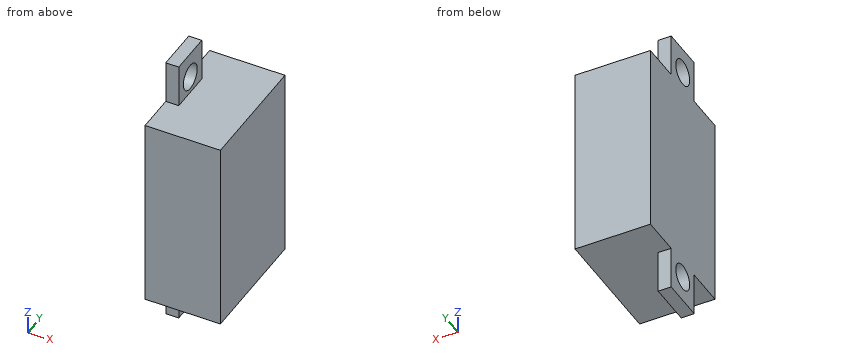
Autodesk Inventor part; units mm, degrees
ref_plane "YZ Plane" through (0, 0, 0) normal (1, 0, 0) x (0, 1, 0)
ref_plane "XZ Plane" through (0, 0, 0) normal (0, 1, 0) x (-1, 0, 0)
ref_plane "XY Plane" through (0, 0, 0) normal (0, 0, 1) x (1, 0, 0)
sketch "Sketch1" plane through (0, 0, 0) normal (1, 0, 0) x (0, 1, 0)
  line L0 (0, 0) -> (14, 0)
  line L1 (14, 0) -> (14, -22.5)
  line L2 (14, -22.5) -> (0, -22.5)
  line L3 (0, -22.5) -> (0, 0)
  dimension "d0" = 14
  dimension "d1" = 22.5
extrude "Extrusion1" add sketch "Sketch1" along normal blind 7.2
sketch "Sketch2" plane through (0, 0, 0) normal (-1, 0, 0) x (0, 0, 1)
  line L0 (-22.5, 0) -> (-22.5, 14)
  line L1 (0, 0) -> (-22.5, 0)
  line L2 (0, 14) -> (0, 0)
  line L3 (-22.5, 14) -> (0, 14)
extrude "Extrusion2" add sketch "Sketch2" along normal blind 1.5
sketch "Sketch3" plane through (7.2, 0, 0) normal (0, 0, 1) x (1, 0, 0)
  line L0 (-8.7, 0) -> (-8.7, 14)
  line L1 (-8.7, 14) -> (0, 14)
  line L2 (-8.7, 0) -> (-7.2, 0)
  line L3 (-7.2, 0) -> (-7.2, 14)
  line L4 (-7.2, 14) -> (-8.7, 14)
  line L5 (-8.7, 14) -> (-8.7, 0)
  line L6 (-8.7, 7) -> (-7.2, 7)
  line L7 (-8.7, 9.5) -> (-7.2, 9.5)
  line L8 (-7.2, 9.5) -> (-7.2, 4.5)
  line L9 (-7.2, 4.5) -> (-8.7, 4.5)
  line L10 (-8.7, 4.5) -> (-8.7, 9.5)
  line L11 (-8.7, 9.5) -> (-7.2, 4.5) construction
  line L12 (-7.2, 9.5) -> (-8.7, 4.5) construction
  point P0 (-7.95, 7)
  dimension "d6" = 5
extrude "Extrusion3" add sketch "Sketch3" along normal blind 5 contours L0 L6 L3 L9 | L0 L7 L3 L6
sketch "Sketch4" plane through (7.2, 0, -22.5) normal (0, 0, -1) x (-1, 0, 0)
  line L0 (8.7, 9.5) -> (8.7, 4.5)
  line L1 (8.7, 4.5) -> (7.2, 4.5)
  line L2 (7.2, 4.5) -> (7.2, 9.5)
  line L3 (7.2, 9.5) -> (8.7, 9.5)
  point P0 (7.2, 0)
extrude "Extrusion4" add sketch "Sketch4" along normal blind 5
sketch "Sketch5" plane through (0, 4.5, -22.5) normal (1, 0, 0) x (0, 0, -1)
  line L0 (-22.5, 5) -> (-27.5, 5)
  line L1 (-22.5, 0) -> (-27.5, 0)
  line L2 (-27.5, 0) -> (-27.5, 5)
  line L3 (0, -4.5) -> (0, 9.5)
  line L4 (-22.5, 9.5) -> (-22.5, -4.5)
  line L5 (0, 5) -> (5, 5)
  line L6 (0, 0) -> (5, 0)
  line L7 (-27.5, 2.5) -> (-22.5, 2.5)
  line L8 (0, 2.5) -> (5, 2.5)
  line L9 (-22.5, 2.5) -> (-23, 2.5)
  line L10 (0, 2.5) -> (0.5, 2.5)
  line L11 (-23, 2.5) -> (-24.5, 2.5)
  circle A0 centre (-24.5, 2.5) radius 1.5
  line L12 (0.5, 2.5) -> (2, 2.5)
  circle A1 centre (2, 2.5) radius 1.5
  dimension "d11" = 0.5
  dimension "d12" = 0.5
  dimension "d13" = 1.5
  dimension "d14" = 1.5
extrude "Extrusion5" cut sketch "Sketch5" against normal blind 5 contours A0 L7 | L7 A0 | A1 L8 | L8 A1
sketch "Sketch6" plane through (7.2, 0, 0) normal (1, 0, 0) x (0, 0, -1)
  line L0 (0, 14) -> (22.5, 14)
  line L1 (0, 14) -> (22.6011, 13.9799) construction
  line L2 (22.6011, 13.9799) -> (22.5897, 1.2087) construction
  line L3 (22.5897, 1.2087) -> (-0.0114, 1.2289) construction
  line L4 (-0.0114, 1.2289) -> (0, 14) construction
  point P0 (0, 0)
properties part number "Voltmeter"
Design review of the part built by this model. Coordinates are the model's own, in mm. Give positions to 0.01 mm unless a question says otherwise; leave off trailing zeros. Order: outer loops, then holes, each group sorted by start corner. A loop starts at its lowest first (then second) coordinate and runs counter-clockwise, first axis right, second up. Notation, with made-up numbers: (33.5, 57) - (40.5, 57) arc R23 cw to (40.5, 85) - close; hole circle Ø4 at (58.25, -31.5). An arc over 180 degrees is marked (long way). Write item = value, one per line. Start each with the question number.
Q1. To check wall thickness, follow L1, parallel to Z at x = -0.6, y = 7; L2, parallel to Y at x = -0.85, z = -24.5; L3, parallel to Z at x = 4.75, y = 13. State the ranges of each line that lie inside material, in increasing order. Write a range as from..to.
Q2. We need section B-B on z = -24.5. State the section outline as (x, y) points, plus the area to 3 significant figures.
Q3. We need section A-A on y = 7. State the section outline as (x, z) points.
Q4. Clearance check with flat-ended pins moving along their axes: pin 1 Ø2.5 at (y, z) = (7.5, 2.5) entering from +X; pin 2 Ø2.5 at (y, z) = (7, 2) entering from +X; pin 3 Ø1.2 at (x, z) = (-1, 3) entering from -Y. State where each tip first meets the part, or that it passes through.
Q5. We need section D-D on y = 1.5. State the section outline as (x, z) points.
Q6. We need section C-C on x = 6.5. State the section outline as (y, z) points.
Working result:
q1.L1 = -27.5..-26, -23..0.5, 3.5..5
q1.L2 = 4.5..5.5, 8.5..9.5
q1.L3 = -22.5..0
q2.outline = (-1.5, 4.5) - (0, 4.5) - (0, 5.5) - (-1.5, 5.5) - close; (-1.5, 8.5) - (0, 8.5) - (0, 9.5) - (-1.5, 9.5) - close
q2.area = 3.00 mm²
q3.outline = (-1.5, -27.5) - (0, -27.5) - (0, -26) - (-1.5, -26) - close; (-1.5, -23) - (0, -23) - (0, -22.5) - (7.2, -22.5) - (7.2, 0) - (0, 0) - (0, 0.5) - (-1.5, 0.5) - close; (-1.5, 3.5) - (0, 3.5) - (0, 5) - (-1.5, 5) - close
q4.pin_1 = 0
q4.pin_2 = through
q4.pin_3 = 4.5
q5.outline = (-1.5, -22.5) - (7.2, -22.5) - (7.2, 0) - (-1.5, 0) - close
q6.outline = (0, -22.5) - (14, -22.5) - (14, 0) - (0, 0) - close
